Here's how the part is built. I have some questions about the finished solid (model axes, mm). A direction names the side the tool comes from. Round coordinates to 2 decimals unless told otherwise and drop trailing zeros. Order: outer loops, then holes, each group sorted by start corner. A loop starts at its lowest first (then second) coordinate and runs counter-clockwise, first axis right, second up. Notation, with made-up numbers: (55.5, 81.5) -> (83.5, 81.5) arc R31 ccw to (83.5, 112.5) -> close; hole circle Ø4 at (6, -6). An arc over 180 degrees is marked (long way). Use a Markdown table: item, result. Add a question column.
(1) I want a section at D-D, the plane y = 41.5. Please give me the cut outline in (x, z) (3 decimals), then the cut area to 3 significant figures.
(2) On a 3-axis mill with a long thin cutter (end or side, diameter ignored), from which of +Z, -Z, +X, -X, +Y, -Y can I reach the whole of each face in a straight line? I mean faces 5 (the face through (0, 90, 0)), 6 (the face through (-12, 28, 0)), 7 (the face through (8.03, 36.98, 5.12)). Say none if no direction works.
(3) If I drill on probe 1 along Y at (x, z) = (-15.5, 0); probe 2 along X at (y, z) = (73, -0.5); probe 3 along Z at (x, y) = (-16.5, 68.3), over which ranges is the centre line in solid material (lowest first)?
(4) Thinking about a two-plate mould opening in X: for faces 1 (the face through (-20, 44, 0)), 2 (the face through (20, 44, 0)), 3 (the face through (-14.59, 65.37, -0.65)), 4 (the face through (0, 75, 0)), which applies, pulls with the +X half, pulls with the -X half, needs draft (parallel to the pull), parting line crosses it, or undercut?
(5) I want a section at A-A, the plane z = 0. Please give me the cut outline in (x, y) (3 decimals), then the cut area to 3 significant figures.
(6) I want a section at B-B, the plane x = 0. Please give me the cut outline in (y, z) (3 decimals), then the cut area to 3 significant figures.
(7) I want a section at C-C, the plane y = 68.3. Please give me the cut outline in (x, z) (3 decimals), then the cut area to 3 significant figures.
(8) I'm going to push flat-ended pins straight in: P1, Ø1.5, axis at y = 27.5, z = -1, coming from the -X side; P2, Ø1, axis at x = 0, z = -3.5, coming from the -Y side. Where does each tip first touch, or does it pass through?
from build123d import *

# Parameters (mm, degrees)
SKETCH1_W           = 40
SKETCH1_H           = 40
BOSS_EXTRUDE1_DEPTH = 90
SKETCH2_R           = 9.525
CUT_EXTRUDE1_DEPTH  = 75
SKETCH3_R           = 3
CUT_EXTRUDE5_DEPTH  = 17
SKETCH5_R           = 2.5
CUT_EXTRUDE6_DEPTH  = 8


with BuildPart() as part:
    # Sketch1 → Boss-Extrude1 (new body)
    with BuildSketch(Plane(origin=(0, 0, 0), x_dir=(1, 0, 0), z_dir=(0, 1, 0))):
        Rectangle(SKETCH1_W, SKETCH1_H)
    extrude(amount=BOSS_EXTRUDE1_DEPTH)

    # Sketch2 → Cut-Extrude1 (cut)
    with BuildSketch(Plane(origin=(0, 0, 0), x_dir=(1, 0, 0), z_dir=(0, 1, 0))):
        with Locations(Location((0, 0, 0), (0, 0, 270))):
            Circle(SKETCH2_R)
    extrude(amount=CUT_EXTRUDE1_DEPTH, mode=Mode.SUBTRACT)

    # Sketch3 → Cut-Extrude5 (cut)
    with BuildSketch(Plane.ZY.offset(20)):
        with Locations((0, 68.3)):
            Circle(SKETCH3_R)
    extrude(amount=-CUT_EXTRUDE5_DEPTH, mode=Mode.SUBTRACT)

    # Sketch5 → Cut-Extrude6 (cut)
    with BuildSketch(Plane.ZY.offset(20)):
        with Locations((0, 27.5)):
            Circle(SKETCH5_R)
    extrude(amount=-CUT_EXTRUDE6_DEPTH, mode=Mode.SUBTRACT)


solid = part.part
Taken from the geometry:
| question | item | result |
|---|---|---|
| 1 | outline | (-20, -20) -> (20, -20) -> (20, 20) -> (-20, 20) -> close; hole circle Ø19.05 at (0, 0) |
| 1 | area | 1,310 mm2 |
| 2 | face 5 | +Z, -Z, +X, -X, +Y |
| 2 | face 6 | -X |
| 2 | face 7 | -Y |
| 3 | probe 1 | y = 0 to 25, 30 to 65.3, 71.3 to 90 |
| 3 | probe 2 | x = -20 to -9.51, 9.51 to 20 |
| 3 | probe 3 | z = -20 to -3, 3 to 20 |
| 4 | face 1 | pulls with the -X half |
| 4 | face 2 | pulls with the +X half |
| 4 | face 3 | needs draft |
| 4 | face 4 | undercut |
| 5 | outline | (-20, 0) -> (-9.525, 0) -> (-9.525, 65.3) -> (-20, 65.3) -> (-20, 30) -> (-12, 30) -> (-12, 25) -> (-20, 25) -> close; (-20, 71.3) -> (-9.525, 71.3) -> (-9.525, 75) -> (9.525, 75) -> (9.525, 0) -> (20, 0) -> (20, 90) -> (-20, 90) -> close |
| 5 | area | 2,070 mm2 |
| 6 | outline | (0, -20) -> (90, -20) -> (90, 20) -> (0, 20) -> (0, 9.525) -> (75, 9.525) -> (75, -9.525) -> (0, -9.525) -> close |
| 6 | area | 2,170 mm2 |
| 7 | outline | (-20, -20) -> (20, -20) -> (20, 20) -> (-20, 20) -> (-20, 3) -> (-9.04, 3) arc R9.525 cw (long way) to (-9.04, -3) -> (-20, -3) -> close |
| 7 | area | 1,250 mm2 |
| 8 | P1 | stops at x = -12 |
| 8 | P2 | stops at y = 75 |
